```python
from build123d import *

# Parameters (mm, degrees)
F0_W     = 102.1404191852
F0_H     = 101.830907166
F1_DEPTH = 101.6
F2_DEPTH = 25.4
F3_R     = 25.4
F4_DEPTH = 101.6
F7_W     = 50.8
F7_H     = 50.8
F8_DEPTH = 101.6
F9_R     = 5.08


with BuildPart() as f1:
    # F0 (on Top) → F1 (new body)
    with BuildSketch(Plane.XY):
        Rectangle(F0_W, F0_H)
    extrude(amount=F1_DEPTH)

    # F2 (add): a face of the model
    f2_faces = [f1.faces().sort_by_distance(p)[0] for p in [
        (0, 0, 101.6),
    ]]
    extrude(f2_faces, amount=F2_DEPTH)

    # F3 (on face) → F4 (join)
    with BuildSketch(Plane.XY.offset(127)):
        Circle(F3_R)
    extrude(amount=F4_DEPTH)

    # F5 (on face) → F6 (revolve)
    with BuildSketch(Plane.XY.offset(228.6)):
        with BuildLine():
            Line((0, -25.4), (0, -38.1))
            ThreePointArc((0, -38.1), (38.1, 0), (0, 38.1))
            Line((0, 38.1), (0, 25.4))
            ThreePointArc((0, 25.4), (17.9605122421, 17.9605122421), (25.4, 0))
            ThreePointArc((25.4, 0), (17.9605122421, -17.9605122421), (0, -25.4))
        make_face()
    revolve(axis=Axis((0, 0, 228.6), (0, -1, 0)))

    # F7 (on face) → F8 (cut)
    with BuildSketch(Plane.YZ.offset(51.0702095926)):
        with Locations((0, 61.0084416688)):
            Rectangle(F7_W, F7_H)
    extrude(amount=-F8_DEPTH, mode=Mode.SUBTRACT)

    # F9
    f9_edges = [f1.edges().sort_by_distance(p)[0] for p in [
        (0, 50.915454, 127),
        (51.07021, 50.915454, 63.5),
        (-51.07021, 50.915454, 63.5),
        (0, 50.915454, 0),
        (51.07021, 0, 127),
        (51.07021, -50.915454, 63.5),
        (51.07021, 0, 0),
        (51.07021, 0, 86.408442),
        (51.07021, 25.4, 61.008442),
        (51.07021, 0, 35.608442),
        (51.07021, -25.4, 61.008442),
        (-51.07021, 0, 0),
        (0, -50.915454, 0),
        (0, -50.915454, 127),
        (-51.07021, 0, 127),
        (-51.07021, -50.915454, 63.5),
        (-25.4, 0, 200.201937),
        (-25.4, 0, 127),
        (25.4, 0, 163.600968),
    ]]
    fillet(f9_edges, radius=F9_R)


solid = f1.part
```
Geometry check sheet. Reference: the model listing, model coordinates, mm. A direction names the side the tool comes from. Coordinates: 2 decimals unless noted, no trailing zeros. Loops run counter-clockwise (first coordinate to the right, second up) from the corner with the lowest first, then second, coordinate; pieces in that order, holes last. Notation, with made-up numbers: (-39, 35.5) -> (0, 35.5) arc R25 cw to (0, 61.5) -> close; hole circle Ø8 at (50, 79). An arc over 180 degrees is marked (long way). Put each result on its own line as item: value.
1) Gauge pin test, flat ends, axial feed: pin 1 Ø15 at (x, y) = (18, 0.5) entering from +Z; pin 2 Ø5 at (y, z) = (-16, 34) entering from +X; pin 3 Ø5 at (y, z) = (-2, 165) entering from +X; pin 4 Ø10 at (x, z) = (32, 138.5) entering from +Y. Record the tip position at first contact, or that the pin passes through.
Result set:
pin 1: stops at z = 265.22
pin 2: stops at x = 50.98
pin 3: stops at x = 25.4
pin 4: passes through
2) Cross-section at A-A on x = -43. Record the boundary of the cut face in (y, z).
Result set:
outline: (-50.92, 5.08) arc R5.08 ccw to (-45.84, 0) -> (45.84, 0) arc R5.08 ccw to (50.92, 5.08) -> (50.92, 121.92) arc R5.08 ccw to (45.84, 127) -> (-45.84, 127) arc R5.08 ccw to (-50.92, 121.92) -> close; hole (-25.4, 35.61) -> (25.4, 35.61) -> (25.4, 86.41) -> (-25.4, 86.41) -> close
3) Cross-section at D-D on z = 215. Record the boundary of the cut face in (x, y).
Result set:
outline: circle Ø71.18 at (0, 0)
4) Thickness scan on line 1 (Z direction, x = 41, y = 6.5); line 2 (Y direction, x = -9, z = 45.5); line 3 (Z direction, x = 12, y = -16). Record the ranges inside material, lowest first.
Result set:
line 1: z = 0 to 35.61, 86.41 to 127
line 2: y = -50.92 to -25.4, 25.4 to 50.92
line 3: z = 0 to 35.61, 86.41 to 228.6, 244.26 to 261.03
5) Tool access check on faces 1 (the cylindrical face through (-49.62, 49.39, 62.68)), 2 (the flat face through (-50.53, 0, 61)), 3 (the cylindrical face through (-20.157, -15.456, 164.586)). Record the directions out of +Z, -Z, +X, -X, +Y, -Y that give a thin tool (end or side, any length) a straight path to the whole face; none if there is none.
Result set:
face 1: +Z, -Z, -X, +Y
face 2: +X
face 3: none
6) Cross-section at C-C on x = 0. Count the separate pieces of the cut face and the enclosed holes in it, plus the area to 3 significant figures.
Result set:
separate pieces: 1
enclosed holes: 2
area: 17,300 mm^2
7) Cross-section at B-B on z = 42. Record the boundary of the cut face in (x, y), plus the area to 3 significant figures.
Result set:
outline: (-51.07, -45.84) arc R5.08 ccw to (-45.99, -50.92) -> (45.99, -50.92) arc R5.08 ccw to (51.07, -45.84) -> (51.07, -30.48) arc R5.08 ccw to (45.99, -25.4) -> (-50.53, -25.4) -> (-50.53, 25.4) -> (45.99, 25.4) arc R5.08 ccw to (51.07, 30.48) -> (51.07, 45.84) arc R5.08 ccw to (45.99, 50.92) -> (-45.99, 50.92) arc R5.08 ccw to (-51.07, 45.84) -> close
area: 5,210 mm^2
8) Release check for a two-part mould opening along Z. For faces 4 (the flat face through (-1, -50.915, 63)), 5 (the flat face through (-2, -25.4, 61)), 6 (the cylindrical face through (49.622, -26.928, 61.435)), 7 (the cylindrical face through (0.64, 49.39, 125.55)) record: released by +Z, released by -Z, zero draft, split by the parting line, or undercut.
Result set:
face 4: zero draft
face 5: undercut
face 6: undercut
face 7: released by +Z
